Geometry check sheet. Reference: the model listing, model coordinates, mm. Face numbers are marked on the shaded views. Give positions to 0.01 mm unless a question says otherwise; leave off trailing zeros. Loops run counter-clockwise (first coordinate to the right, second up) from the corner with the lowest first, then second, coordinate; pieces in that order, holes last.
1. Go/stop test with a flat-tipped pin: pin 1 Ø2 at (x, y) = (20.5, 6.5) entering from -Z. Record where the tip stops, or that it passes through.
2. Cross-section at B-B, the plane y = 6. Record the cut outline in (x, z), plus the area to 3 significant figures.
3. Cross-section at D-D, the plane y = 4.25. Record the cut outline in (x, z), plus the area to 3 significant figures.
4. Cross-section at C-C, the plane z = 8.25. Record the cut outline in (x, y) (3 decimals).
5. Cross-section at A-A, the plane x = 5. Record the cut outline in (y, z), plus the area to 3 significant figures.
6. Release check for a two-part mould opening along X. For the marked faces 1, 2, 3 and 4 record: +X half, -X half, draft (parallel to the pull), parting line (faces both ways), or undercut.
7. Material ranges on L1, parallel to Y at x = 5, z = 4.25; L2, parallel to X at y = 7.5, z = 7.25; L3, parallel to X at y = 7, z = 9.5, recorded low to high.
Autodesk Inventor part; units mm, degrees
ref_plane "YZ Plane" through (0, 0, 0) normal (1, 0, 0) x (0, 1, 0)
ref_plane "XZ Plane" through (0, 0, 0) normal (0, 1, 0) x (-1, 0, 0)
ref_plane "XY Plane" through (0, 0, 0) normal (0, 0, 1) x (1, 0, 0)
sketch "Sketch1" plane through (0, 0, 0) normal (0, 0, 1) x (1, 0, 0)
  line L0 (27, 1) -> (27, 11)
  line L1 (0, 11) -> (0, 1)
  circle A0 centre (5, 6) radius 3
  circle A1 centre (13.125, 6) radius 3.125
  circle A2 centre (21.5, 6) radius 3.25
  line L2 (0, 11) -> (27, 11)
  line L3 (0, 1) -> (27, 1)
  point P0 (0, 0)
  dimension "d2" = 6
  dimension "d3" = 6.25
  dimension "d4" = 6.5
  dimension "d7" = 8.375
  dimension "d8" = 5
  dimension "d9" = 5
extrude "Extrusion1" add sketch "Sketch1" along normal blind 10
fillet "Fillet1" radius 2 4 edges at (0, 11, 5) (27, 11, 5) (27, 1, 5) (0, 1, 5)
properties part number "6mmHoleTest6-6.25-6.5mm"
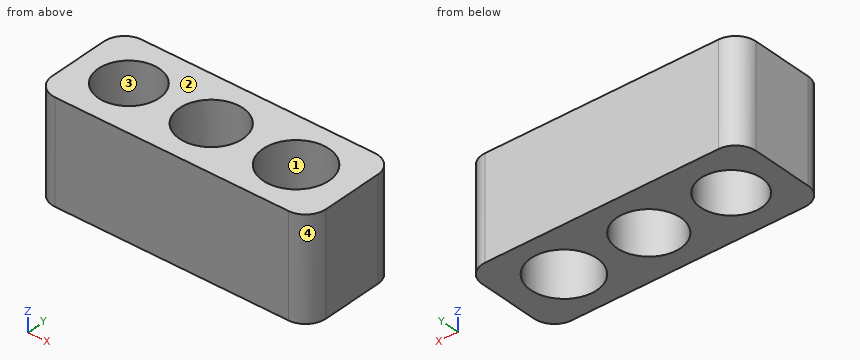
Result:
1. pin 1: passes through
2. outline: (0, 0) - (2, 0) - (2, 10) - (0, 10) - close; (8, 0) - (10, 0) - (10, 10) - (8, 10) - close; (16.25, 0) - (18.25, 0) - (18.25, 10) - (16.25, 10) - close; (24.75, 0) - (27, 0) - (27, 10) - (24.75, 10) - close
2. area: 82.5 mm2
3. outline: (0, 0) - (2.56, 0) - (2.56, 10) - (0, 10) - close; (7.44, 0) - (10.54, 0) - (10.54, 10) - (7.44, 10) - close; (15.71, 0) - (18.76, 0) - (18.76, 10) - (15.71, 10) - close; (24.24, 0) - (27, 0) - (27, 10) - (24.24, 10) - close
3. area: 115 mm2
4. outline: (0, 3) arc R2 ccw to (2, 1) - (25, 1) arc R2 ccw to (27, 3) - (27, 9) arc R2 ccw to (25, 11) - (2, 11) arc R2 ccw to (0, 9) - close; hole circle Ø6 at (5, 6); hole circle Ø6.25 at (13.125, 6); hole circle Ø6.5 at (21.5, 6)
5. outline: (1, 0) - (3, 0) - (3, 10) - (1, 10) - close; (9, 0) - (11, 0) - (11, 10) - (9, 10) - close
5. area: 40.0 mm2
6. face 1: undercut
6. face 2: draft
6. face 3: undercut
6. face 4: +X half
7. L1: y = 1 to 3, 9 to 11
7. L2: x = 0 to 2.4, 7.6 to 10.38, 15.87 to 18.62, 24.38 to 27
7. L3: x = 0 to 2.17, 7.83 to 10.16, 16.09 to 18.41, 24.59 to 27
